Verification items for this drawing (mm, ordinates from the low corner). Round coordinates to 2 decimals unless told otherwise and drop trailing zeros. Write each loop counter-clockwise with the first axis right and the second up, starting at its lowest first coordinate (ties: lowest second). Pieces come first, ordered by that corner, then holes. Notation, with made-up numbers: (-21.75, 5.5) - (36.25, 5.5) arc R22 ccw to (36.25, 37.5) - close; hole circle Ø11 at (-17.5, 87.5). An arc over 180 degrees is marked (long way). One line per question, with ' | ' between items. Start each with the question number.
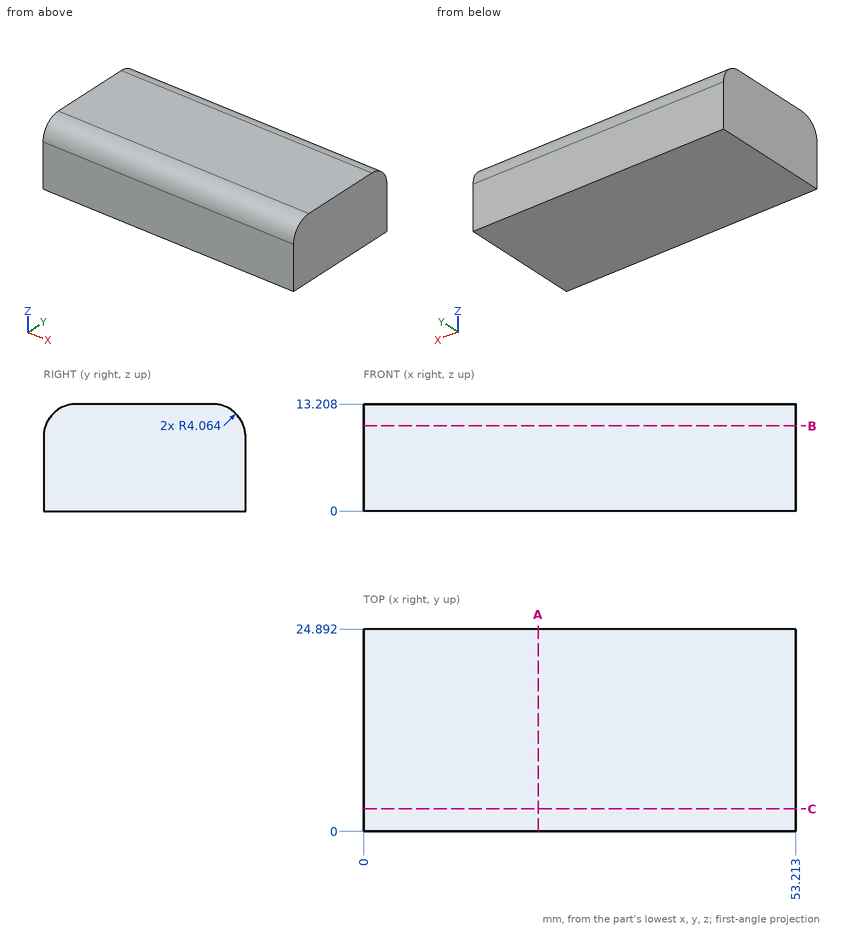
Q1. Thickness scan on line 1 (Y direction, x = 31.5, z = 12); line 2 (Z direction, x = 31, y = 22.75); line 3 (Z direction, x = 20.5, y = 23.5). Record the ranges inside material, lowest first.
Q2. Section check A-A, the plane x = 21.5. Record the cut outline in (y, z).
Q3. Section check C-C, the plane y = 2.75. Record the cut outline in (x, z), then the cut area to 3 significant figures.
Q4. Section check B-B, the plane z = 10.5. Record the cut outline in (x, y).
Result sheet:
1) line 1: 1.17 to 23.72 | line 2: 0 to 12.72 | line 3: 0 to 12.21
2) outline: (0, 0) - (24.89, 0) - (24.89, 9.14) arc R4.06 ccw to (20.83, 13.21) - (4.06, 13.21) arc R4.06 ccw to (0, 9.14) - close
3) outline: (0, 0) - (53.21, 0) - (53.21, 12.99) - (0, 12.99) - close | area: 691 mm²
4) outline: (0, 0.23) - (53.21, 0.23) - (53.21, 24.66) - (0, 24.66) - close
